Verification items for the finished model (mm, model axes). A direction names the side the tool comes from. Coordinates: 2 decimals unless noted, no trailing zeros. Return JSON: item names as keys, results as strings.
```python
from build123d import *

# Parameters (mm, degrees)
F1_DEPTH = 10
F3_DEPTH = 1
F5_DEPTH = 8
F6_R     = 4
F6_R_2   = 2
F7_DEPTH = 10


with BuildPart() as f1:
    # F0 (on Top) → F1 (new body)
    with BuildSketch(Plane.XY):
        with BuildLine():
            ThreePointArc((66, 32), (65.12132, 29.87868), (63, 29))
            Line((63, 29), (6, 29))
            ThreePointArc((6, 29), (3.87868, 29.87868), (3, 32))
            ThreePointArc((3, 32), (0, 35), (-3, 32))
            ThreePointArc((-3, 32), (-3.87868, 29.87868), (-6, 29))
            Line((-6, 29), (-63, 29))
            ThreePointArc((-63, 29), (-65.12132, 29.87868), (-66, 32))
            ThreePointArc((-66, 32), (-69, 35), (-72, 32))
            ThreePointArc((-72, 32), (-72.87868, 29.87868), (-75, 29))
            Line((-75, 29), (-75, -29))
            ThreePointArc((-75, -29), (-72.87868, -29.87868), (-72, -32))
            ThreePointArc((-72, -32), (-69, -35), (-66, -32))
            ThreePointArc((-66, -32), (-65.12132, -29.87868), (-63, -29))
            Line((-63, -29), (-6, -29))
            ThreePointArc((-6, -29), (-3.87868, -29.87868), (-3, -32))
            ThreePointArc((-3, -32), (0, -35), (3, -32))
            ThreePointArc((3, -32), (3.87868, -29.87868), (6, -29))
            Line((6, -29), (63, -29))
            ThreePointArc((63, -29), (65.12132, -29.87868), (66, -32))
            ThreePointArc((66, -32), (69, -35), (72, -32))
            ThreePointArc((72, -32), (72.87868, -29.87868), (75, -29))
            Line((75, -29), (75, 29))
            ThreePointArc((75, 29), (72.87868, 29.87868), (72, 32))
            ThreePointArc((72, 32), (69, 35), (66, 32))
        make_face()
    extrude(amount=-F1_DEPTH)

    # F2 (on face) → F3 (cut)
    with BuildSketch(Plane.XY):
        with BuildLine():
            ThreePointArc((72.5, 21.5), (71.035534, 25.035534), (67.5, 26.5))
            Line((67.5, 26.5), (-67.5, 26.5))
            ThreePointArc((-67.5, 26.5), (-71.035534, 25.035534), (-72.5, 21.5))
            Line((-72.5, 21.5), (-72.5, -21.5))
            ThreePointArc((-72.5, -21.5), (-71.035534, -25.035534), (-67.5, -26.5))
            Line((-67.5, -26.5), (67.5, -26.5))
            ThreePointArc((67.5, -26.5), (71.035534, -25.035534), (72.5, -21.5))
            Line((72.5, -21.5), (72.5, 21.5))
        make_face()
        with BuildLine():
            Line((-67.5, 24.5), (67.5, 24.5))
            ThreePointArc((67.5, 24.5), (69.62132, 23.62132), (70.5, 21.5))
            Line((70.5, 21.5), (70.5, -21.5))
            ThreePointArc((70.5, -21.5), (69.62132, -23.62132), (67.5, -24.5))
            Line((67.5, -24.5), (-67.5, -24.5))
            ThreePointArc((-67.5, -24.5), (-69.62132, -23.62132), (-70.5, -21.5))
            Line((-70.5, -21.5), (-70.5, 21.5))
            ThreePointArc((-70.5, 21.5), (-69.62132, 23.62132), (-67.5, 24.5))
        make_face(mode=Mode.SUBTRACT)
    extrude(amount=-F3_DEPTH, mode=Mode.SUBTRACT)

    # F4 (on face) → F5 (cut)
    with BuildSketch(Plane.XY):
        with BuildLine():
            Line((67, -18.9), (-67, -18.9))
            ThreePointArc((-67, -18.9), (-69.1, -21), (-67, -23.1))
            Line((-67, -23.1), (67, -23.1))
            ThreePointArc((67, -23.1), (68.484924, -22.484924), (69.1, -21))
            Line((69.1, -21), (69.1, -16.4))
            ThreePointArc((69.1, -16.4), (68.484924, -14.915076), (67, -14.3))
            Line((67, -14.3), (-67, -14.3))
            Line((-67, -14.3), (-67, -13.9))
            Line((-67, -13.9), (67, -13.9))
            ThreePointArc((67, -13.9), (68.484924, -13.284924), (69.1, -11.8))
            Line((69.1, -11.8), (69.1, -7.2))
            ThreePointArc((69.1, -7.2), (68.484924, -5.715076), (67, -5.1))
            Line((67, -5.1), (-67, -5.1))
            Line((-67, -5.1), (-67, -4.7))
            Line((-67, -4.7), (67, -4.7))
            ThreePointArc((67, -4.7), (68.484924, -4.084924), (69.1, -2.6))
            Line((69.1, -2.6), (69.1, 2))
            ThreePointArc((69.1, 2), (68.484924, 3.484924), (67, 4.1))
            Line((67, 4.1), (-67, 4.1))
            Line((-67, 4.1), (-67, 4.5))
            Line((-67, 4.5), (67, 4.5))
            ThreePointArc((67, 4.5), (68.484924, 5.115076), (69.1, 6.6))
            Line((69.1, 6.6), (69.1, 11.2))
            ThreePointArc((69.1, 11.2), (68.484924, 12.684924), (67, 13.3))
            Line((67, 13.3), (-67, 13.3))
            Line((-67, 13.3), (-67, 13.7))
            Line((-67, 13.7), (67, 13.7))
            ThreePointArc((67, 13.7), (68.484924, 14.315076), (69.1, 15.8))
            Line((69.1, 15.8), (69.1, 20.4))
            ThreePointArc((69.1, 20.4), (68.484924, 21.884924), (67, 22.5))
            Line((67, 22.5), (-67, 22.5))
            ThreePointArc((-67, 22.5), (-69.1, 20.4), (-67, 18.3))
            Line((-67, 18.3), (67, 18.3))
            Line((67, 18.3), (67, 17.9))
            Line((67, 17.9), (-67, 17.9))
            ThreePointArc((-67, 17.9), (-68.484924, 17.284924), (-69.1, 15.8))
            Line((-69.1, 15.8), (-69.1, 11.2))
            ThreePointArc((-69.1, 11.2), (-68.484924, 9.715076), (-67, 9.1))
            Line((-67, 9.1), (67, 9.1))
            Line((67, 9.1), (67, 8.7))
            Line((67, 8.7), (-67, 8.7))
            ThreePointArc((-67, 8.7), (-68.484924, 8.084924), (-69.1, 6.6))
            Line((-69.1, 6.6), (-69.1, 2))
            ThreePointArc((-69.1, 2), (-68.484924, 0.515076), (-67, -0.1))
            Line((-67, -0.1), (67, -0.1))
            Line((67, -0.1), (67, -0.5))
            Line((67, -0.5), (-67, -0.5))
            ThreePointArc((-67, -0.5), (-68.484924, -1.115076), (-69.1, -2.6))
            Line((-69.1, -2.6), (-69.1, -7.2))
            ThreePointArc((-69.1, -7.2), (-68.484924, -8.684924), (-67, -9.3))
            Line((-67, -9.3), (67, -9.3))
            Line((67, -9.3), (67, -9.7))
            Line((67, -9.7), (-67, -9.7))
            ThreePointArc((-67, -9.7), (-68.484924, -10.315076), (-69.1, -11.8))
            Line((-69.1, -11.8), (-69.1, -16.4))
            ThreePointArc((-69.1, -16.4), (-68.484924, -17.884924), (-67, -18.5))
            Line((-67, -18.5), (67, -18.5))
            Line((67, -18.5), (67, -18.9))
        make_face()
    extrude(amount=-F5_DEPTH, mode=Mode.SUBTRACT)

    # F6 (on face) → F7 (join)
    with BuildSketch(Plane(origin=(-75, 0, 0), x_dir=(0, -1, 0), z_dir=(-1, 0, 0))):
        with Locations((-20.4, -4)):
            Circle(F6_R)
        with Locations((-20.4, -4)):
            Circle(F6_R_2, mode=Mode.SUBTRACT)
        with Locations((21, -4)):
            Circle(F6_R)
        with Locations((21, -4)):
            Circle(F6_R_2, mode=Mode.SUBTRACT)
    extrude(amount=F7_DEPTH)


solid = f1.part
```
Q1. Draft check along Y on faces 1 (the face through (35, 29, -5)), 2 (the face through (75, 0, -5)), 3 (the face through (-71, 25.07, -0.49)). Enter one of: pulls with the +Y half, pulls with the -Y half, needs draft (parallel to the pull), parting line crosses it, or undercut.
Values:
{"face 1": "pulls with the +Y half", "face 2": "needs draft", "face 3": "undercut"}
Q2. Tool access check on faces 4 (the face through (-6, 24, 0)), 5 (the face through (-79.93, 18.492, -3.399)), 6 (the face through (-1, -23.1, -4)). Record the directions out of +Z, -Z, +X, -X, +Y, -Y that give a thin tool (end or side, any length) a straight path to the whole face; none if there is none.
Values:
{"face 4": "+Z, +X, -X, +Y, -Y", "face 5": "-X", "face 6": "+Z"}
Q3. Material ranges on line 1 along X through (y, z) = (20.5, -0.75); line 2 along X through (y, z) = (32, -0.25); line 3 along Z through (x, y) = (-82.5, 20.4), recorded low to high.
Values:
{"line 1": "-85 to -72.5, -70.5 to -69.1, 69.1 to 70.5, 72.5 to 75", "line 2": "-72 to -66, -3 to 3, 66 to 72", "line 3": "-8 to -6, -2 to 0"}
Q4. Go/stop test with flat-tipped pins: pin 1 (3 mm diameter, centred on y = -3, z = -7.5, fed in from -X); pin 2 (0.8 mm diameter, centred on x = 7.5, z = -0.5, fed in from -Y); pin 3 (3 mm diameter, centred on x = 44, z = -5.5, fed in from +Y). Record where each tip stops, or that it passes through.
Values:
{"pin 1": "x = -75", "pin 2": "y = -29", "pin 3": "y = 29"}
